Geometry: final body of the model. Coordinates: model frame, mm. Give positions to 0.01 mm unless a question says otherwise; leave off trailing zeros. Write each loop counter-clockwise with the first axis right and the second up, starting at its lowest first coordinate (ties: lowest second). Pieces come first, ordered by that corner, then holes. Notation, with made-up numbers: (59, 23.25) -> (105, 23.25) arc R29 ccw to (105, 50.25) -> close; hole circle Ø4 at (20, 38.25). An arc over 180 degrees is marked (long way). Use CSV: the item, a comma, the result in double quotes. Start each with the question number.
1) Draft query along Z for faces 1 (the face through (0, 5, -4)), 2 (the face through (35, 5, -7.75)), 3 (the face through (66.57, 4.94, -1.92)). Return one class per face: pulls with the +Z half, pulls with the -Z half, needs draft (parallel to the pull), parting line crosses it, or undercut.
2) Section B-B (y = 8). Output: boundary loops of the cut face in (x, z) (3 decimals).
3) Section A-A (x = 67). Output: boundary loops of the cut face in (y, z) (3 decimals).
4) Material intervals for line 1 (Z direction, x = 3, y = 5.75) (3 decimals); line 2 (X direction, y = 1.5, z = -2.75); line 3 (X direction, y = 0.75, z = -2.25), sorted ascending. Write a range as [from, to].
```python
from build123d import *

# Parameters (mm, degrees)
SKETCH1_W           = 7.75
SKETCH1_H           = 9.75
BOSS_EXTRUDE1_DEPTH = 70
SKETCH4_R           = 2
CUT_EXTRUDE3_DEPTH  = 9.75
CHAMFER1_SIZE       = 0.5
CHAMFER2_SIZE       = 0.5


with BuildPart() as part:
    # Sketch1 → Boss-Extrude1 (new body)
    with BuildSketch(Plane(origin=(0, 0, 0), x_dir=(0, 0, -1), z_dir=(1, 0, 0))):
        with Locations((3.875, 4.875)):
            Rectangle(SKETCH1_W, SKETCH1_H)
    extrude(amount=BOSS_EXTRUDE1_DEPTH)

    # Sketch4 → Cut-Extrude3 (cut)
    with BuildSketch(Plane(origin=(0, 9.75, 0), x_dir=(1, 0, 0), z_dir=(0, 1, 0))):
        with Locations((3, 3.875)):
            Circle(SKETCH4_R)
        with Locations((67, 3.875)):
            Circle(SKETCH4_R)
    extrude(amount=-CUT_EXTRUDE3_DEPTH, mode=Mode.SUBTRACT)

    # Chamfer1
    chamfer1_edges = [part.edges().sort_by_distance(p)[0] for p in [
        (70, 4.875, -7.75),
        (70, 9.75, -3.875),
        (70, 4.875, 0),
        (0, 9.75, -3.875),
        (0, 4.875, -7.75),
        (0, 0, -3.875),
        (0, 4.875, 0),
        (70, 0, -3.875),
    ]]
    chamfer(chamfer1_edges, length=CHAMFER1_SIZE)

    # Chamfer2
    chamfer2_edges = [part.edges().sort_by_distance(p)[0] for p in [
        (35, 0, -7.75),
        (35, 0, 0),
        (35, 9.75, -7.75),
        (35, 9.75, 0),
    ]]
    chamfer(chamfer2_edges, length=CHAMFER2_SIZE)


solid = part.part
```
Answers follow:
1,face 1,"needs draft"
1,face 2,"pulls with the -Z half"
1,face 3,"undercut"
2,outline,"(0, -7.25) -> (0.5, -7.75) -> (69.5, -7.75) -> (70, -7.25) -> (70, -0.5) -> (69.5, 0) -> (0.5, 0) -> (0, -0.5) -> close; hole circle Ø4 at (3, -3.875); hole circle Ø4 at (67, -3.875)"
3,outline,"(0, -7.25) -> (0.5, -7.75) -> (9.25, -7.75) -> (9.75, -7.25) -> (9.75, -5.875) -> (0, -5.875) -> close; (0, -1.875) -> (9.75, -1.875) -> (9.75, -0.5) -> (9.25, 0) -> (0.5, 0) -> (0, -0.5) -> close"
4,line 1,"z = [-7.75, -5.875], [-1.875, 0]"
4,line 2,"x = [0, 1.35], [4.65, 65.35], [68.65, 70]"
4,line 3,"x = [0, 1.83], [4.17, 65.83], [68.17, 70]"
